```python
from build123d import *

# Parameters (mm, degrees)
CROQUIS2_R                 = 12.5
CROQUIS2_R_2               = 9.5
SALIENTE_EXTRUIR1_DEPTH    = 24
CORTAR_EXTRUIR3_DEPTH      = 191.437747955
CORTAR_EXTRUIR3_DEPTH_BACK = 191.437747955
CROQUIS5_W                 = 8
CROQUIS5_H                 = 49.434743854
CORTAR_EXTRUIR4_DEPTH      = 191.437747955
CORTAR_EXTRUIR4_DEPTH_BACK = 191.437747955
CROQUIS6_W                 = 12
CROQUIS6_H                 = 30
CORTAR_EXTRUIR5_DEPTH      = 159.265939688
CORTAR_EXTRUIR5_DEPTH_BACK = 159.265939688
CROQUIS7_W                 = 14.533349016
CROQUIS7_H                 = 8
REDONDEO1_R                = 4


with BuildPart() as part:
    # Croquis2 → Saliente-Extruir1 (new body)
    # profile 1 of 4: a face of its own
    with BuildSketch(Plane.XY):
        with Locations((-37.533349016, 172.653405471)):
            Circle(CROQUIS2_R)
        with Locations((-37.533349016, 172.653405471)):
            Circle(CROQUIS2_R_2, mode=Mode.SUBTRACT)
    # profile 2 of 4: a face of its own
    with BuildSketch(Plane.XY):
        with BuildLine():
            Line((-12.5, 58.855421297), (-12.5, 0))
            ThreePointArc((-12.5, 0), (0, 12.5), (12.5, 0))
            Line((12.5, 0), (12.5, 115))
            ThreePointArc((12.5, 115), (0.265693313, 156.217157525), (-32.475079629, 184.08423706))
            ThreePointArc((-32.475079629, 184.08423706), (-27.057701844, 179.473289366), (-25.033349016, 172.653405471))
            ThreePointArc((-25.033349016, 172.653405471), (-30.713465121, 162.1777583), (-42.591618403, 161.222573883))
            ThreePointArc((-42.591618403, 161.222573883), (-27.406897086, 150.843693068), (-16.941222141, 135.718661617))
            ThreePointArc((-16.941222141, 135.718661617), (-17.037727548, 131.417260647), (-20.439743892, 128.783319041))
            Line((-20.439743892, 128.783319041), (-27.655370554, 127.214704549))
            ThreePointArc((-27.655370554, 127.214704549), (-17.155961879, 124.732474812), (-12.5, 115))
            ThreePointArc((-12.5, 115), (-16.161165235, 106.161165235), (-25, 102.5))
            Line((-25, 102.5), (-17.5, 102.5))
            ThreePointArc((-17.5, 102.5), (-13.964466094, 101.035533906), (-12.5, 97.5))
            Line((-12.5, 97.5), (-12.5, 58.855421297))
        make_face()
    # profile 3 of 4: a face of its own
    with BuildSketch(Plane.XY):
        with Locations((-25, 115)):
            Circle(CROQUIS2_R)
        with Locations((-25, 115)):
            Circle(CROQUIS2_R_2, mode=Mode.SUBTRACT)
    # profile 4 of 4: a face of its own
    with BuildSketch(Plane.XY):
        Circle(CROQUIS2_R)
        Circle(CROQUIS2_R_2, mode=Mode.SUBTRACT)
    extrude(amount=SALIENTE_EXTRUIR1_DEPTH)

    # Croquis5 → Cortar-Extruir3 (cut, two sides: drawn at the far end of the back side and taken through both)
    with BuildSketch(Plane.ZY.offset(12.5).offset(-CORTAR_EXTRUIR3_DEPTH_BACK)):
        with Locations((12, 160.436033544)):
            Rectangle(CROQUIS5_W, CROQUIS5_H)
    extrude(amount=CORTAR_EXTRUIR3_DEPTH + CORTAR_EXTRUIR3_DEPTH_BACK, mode=Mode.SUBTRACT)

    # Croquis6 → Cortar-Extruir4 (cut, two sides: drawn at the far end of the back side and taken through both)
    with BuildSketch(Plane.ZY.offset(12.5).offset(-CORTAR_EXTRUIR4_DEPTH_BACK)):
        with Locations((12, 2.5)):
            Rectangle(CROQUIS6_W, CROQUIS6_H)
    extrude(amount=CORTAR_EXTRUIR4_DEPTH + CORTAR_EXTRUIR4_DEPTH_BACK, mode=Mode.SUBTRACT)

    # Croquis7 → Cortar-Extruir5 (cut, two sides: drawn at the far end of the back side and taken through both)
    with BuildSketch(Plane(origin=(0, 135.718661617, 0), x_dir=(1, 0, 0), z_dir=(0, 1, 0)).offset(-CORTAR_EXTRUIR5_DEPTH_BACK)):
        with Locations((-42.766674508, -12)):
            Rectangle(CROQUIS7_W, CROQUIS7_H)
    extrude(amount=CORTAR_EXTRUIR5_DEPTH + CORTAR_EXTRUIR5_DEPTH_BACK, mode=Mode.SUBTRACT)

    # Redondeo1
    # the kernel refuses this fillet: 4 mm, written as the material it adds along each edge
    with BuildSketch(Plane(origin=(-26.941222141, 135.718661617, 16), x_dir=(0, 1, 0), z_dir=(1, 0, 0))) as redondeo1_piece_1_section:
        with BuildLine():
            CenterArc((REDONDEO1_R, -REDONDEO1_R), REDONDEO1_R, 90, 90)
            Line((0, -REDONDEO1_R), (-REDONDEO1_R * 0.02, -REDONDEO1_R))
            Line((-REDONDEO1_R * 0.02, -REDONDEO1_R), (-REDONDEO1_R * 0.02, REDONDEO1_R * 0.02))
            Line((-REDONDEO1_R * 0.02, REDONDEO1_R * 0.02), (REDONDEO1_R, REDONDEO1_R * 0.02))
            Line((REDONDEO1_R, REDONDEO1_R * 0.02), (REDONDEO1_R, 0))
        make_face()
    redondeo1_piece_1 = extrude(amount=46.544739715, mode=Mode.PRIVATE)
    redondeo1_piece_1 = redondeo1_piece_1 & Plane(origin=(-63.045397247, 115.0005, 15.097345218), x_dir=(0.9999999999780976, -6.618536910383344e-06, 0), z_dir=(0, 0, -1)) * Cylinder(75.545397249, 110, mode=Mode.PRIVATE)
    redondeo1_piece_1 = redondeo1_piece_1 - Plane(origin=(-63.045397247, 115.0005, 15.097345218), x_dir=(0.40466155096197987, 0.9144665270927335, 0), z_dir=(0, 0, -1)) * Cylinder(50.545397249, 110, mode=Mode.PRIVATE)
    add(redondeo1_piece_1)
    with BuildSketch(Plane(origin=(19.603517574, 135.718661617, 8), x_dir=(0, 0, 1), z_dir=(-1, 0, 0))) as redondeo1_piece_2_section:
        with BuildLine():
            CenterArc((REDONDEO1_R, REDONDEO1_R), REDONDEO1_R, 180, 90)
            Line((0, REDONDEO1_R), (-REDONDEO1_R * 0.02, REDONDEO1_R))
            Line((-REDONDEO1_R * 0.02, REDONDEO1_R), (-REDONDEO1_R * 0.02, -REDONDEO1_R * 0.02))
            Line((-REDONDEO1_R * 0.02, -REDONDEO1_R * 0.02), (REDONDEO1_R, -REDONDEO1_R * 0.02))
            Line((REDONDEO1_R, -REDONDEO1_R * 0.02), (REDONDEO1_R, 0))
        make_face()
    redondeo1_piece_2 = extrude(amount=46.544739715, mode=Mode.PRIVATE)
    redondeo1_piece_2 = redondeo1_piece_2 - Plane(origin=(-63.045397247, 115.0005, 8.902651886), x_dir=(0.40466155096197987, 0.9144665270927335, 0), z_dir=(0, 0, -1)) * Cylinder(50.545397249, 110, mode=Mode.PRIVATE)
    redondeo1_piece_2 = redondeo1_piece_2 & Plane(origin=(-63.045397247, 115.0005, 8.902651886), x_dir=(0.9999999999780976, -6.618536910383344e-06, 0), z_dir=(0, 0, -1)) * Cylinder(75.545397249, 110, mode=Mode.PRIVATE)
    add(redondeo1_piece_2)
    with BuildSketch(Plane(origin=(-12.5, 17.5, 6), x_dir=(0, 0, 1), z_dir=(1, 0, 0))) as redondeo1_piece_3:
        with BuildLine():
            CenterArc((REDONDEO1_R, REDONDEO1_R), REDONDEO1_R, 180, 90)
            Line((0, REDONDEO1_R), (-REDONDEO1_R * 0.02, REDONDEO1_R))
            Line((-REDONDEO1_R * 0.02, REDONDEO1_R), (-REDONDEO1_R * 0.02, -REDONDEO1_R * 0.02))
            Line((-REDONDEO1_R * 0.02, -REDONDEO1_R * 0.02), (REDONDEO1_R, -REDONDEO1_R * 0.02))
            Line((REDONDEO1_R, -REDONDEO1_R * 0.02), (REDONDEO1_R, 0))
        make_face()
    extrude(amount=25)
    with BuildSketch(Plane(origin=(12.5, 17.5, 18), x_dir=(0, -1, 0), z_dir=(-1, 0, 0))) as redondeo1_piece_4:
        with BuildLine():
            CenterArc((REDONDEO1_R, -REDONDEO1_R), REDONDEO1_R, 90, 90)
            Line((0, -REDONDEO1_R), (-REDONDEO1_R * 0.02, -REDONDEO1_R))
            Line((-REDONDEO1_R * 0.02, -REDONDEO1_R), (-REDONDEO1_R * 0.02, REDONDEO1_R * 0.02))
            Line((-REDONDEO1_R * 0.02, REDONDEO1_R * 0.02), (REDONDEO1_R, REDONDEO1_R * 0.02))
            Line((REDONDEO1_R, REDONDEO1_R * 0.02), (REDONDEO1_R, 0))
        make_face()
    extrude(amount=25)


solid = part.part
```
The model under review builds one solid part; all positions refer to its coordinate system, in mm. A direction names the side the tool comes from. Coordinates: 2 decimals unless noted, no trailing zeros. Write each loop counter-clockwise with the first axis right and the second up, starting at its lowest first coordinate (ties: lowest second). Pieces come first, ordered by that corner, then holes. Notation, with made-up numbers: (-20, 78.5) - (34, 78.5) arc R22 ccw to (34, 108.5) - close; hole circle Ø10 at (-2.5, 8.5). An arc over 180 degrees is marked (long way). Write item = value, one per line.
(1) For P1, Ø8, axis at x = -11, z = 17.5, coming from the -Y side; P2, Ø22, axis at x = -37.53, y = 172.65, coming from the +Z side; P3, Ø2, axis at x = -16, z = 10, coming from the -Y side; P4, Ø1.5, axis at x = -39, z = 16.5, coming from the +Y side, all flat-tipped, find the tip position at first contact; note any pin that passes through.
Result sheet:
P1 = -10.33
P2 = 24
P3 = 101.83
P4 = 185.13
(2) Machinability: for faces 5 (the face through (-21, 102.5, 12)), 6 (the face through (-20, 162, 16)), 7 (the face through (-24, 128.01, 11.83)), which of the approach directions +Z, -Z, +X, -X, +Y, -Y give a long, thin tool a straight path to every point of the face, cutting with its end or side? Answer none if there is none.
Result sheet:
face_5 = +Z, -Z, -X, -Y
face_6 = +X, -X, +Y
face_7 = +Z, -Z, -X
(3) For line 1 (Y direction, x = -24, z = 7.75); line 2 (Z direction, x = -27.5, y = 164); line 3 (X direction, y = 32.5, z = 20), list the stretches that pass through material, from the lowest coordinate up. Write a range as [from, to].
Result sheet:
line_1 = [102.5, 105.55], [124.45, 128.01], [147.1, 179.67]
line_2 = [0, 8], [16, 24]
line_3 = [-12.5, 12.5]
(4) Mouldability with a two-part tool opening along X and no side actions: class faces 1 (the face through (-27.591, 151.026, 3.249)), 2 (the face through (4.38, -8.43, 20.96)), 3 (the face through (-5, 9, 18)), 4 (the face through (12.5, 57, 12)) as pulls with the +X half, pulls with the -X half, needs draft (parallel to the pull), parting line crosses it, or undercut.
Result sheet:
face_1 = pulls with the -X half
face_2 = undercut
face_3 = needs draft
face_4 = pulls with the +X half
(5) Consider section A-A, the plane y = 3.5. Give the boundary of the cut face in (x, z).
Result sheet:
outline = (-12.5, 0) - (-8.83, 0) - (-8.83, 6) - (-12.5, 6) - close; (-12.5, 18) - (-8.83, 18) - (-8.83, 24) - (-12.5, 24) - close; (8.83, 0) - (12.5, 0) - (12.5, 6) - (8.83, 6) - close; (8.83, 18) - (12.5, 18) - (12.5, 24) - (8.83, 24) - close
(6) Consider section D-D, the plane z = 20.25. Give the boundary of the cut face in (x, y).
Result sheet:
outline = (-42.59, 161.22) arc R50.55 cw to (-16.94, 135.72) arc R5 cw to (-20.44, 128.78) - (-27.66, 127.21) arc R12.5 ccw to (-25, 102.5) - (-17.5, 102.5) arc R5 cw to (-12.5, 97.5) - (-12.5, 0) arc R12.5 ccw to (12.5, 0) - (12.5, 115) arc R75.55 ccw to (-32.48, 184.08) arc R12.5 ccw to start; hole circle Ø19 at (-37.53, 172.65); hole circle Ø19 at (-25, 115); hole circle Ø19 at (0, 0)
(7) Consider section C-C, the plane x = -45. Give the boundary of the cut face in (y, z), then the cut area to 3 significant figures.
Result sheet:
outline = (162.63, 0) - (166.78, 0) - (166.78, 8) - (162.63, 8) - close; (162.63, 16) - (166.78, 16) - (166.78, 24) - (162.63, 24) - close; (178.53, 0) - (182.68, 0) - (182.68, 8) - (178.53, 8) - close; (178.53, 16) - (182.68, 16) - (182.68, 24) - (178.53, 24) - close
area = 133 mm^2
(8) Consider section B-B, the plane x = 0. Give the boundary of the cut face in (y, z), then the cut area to 3 significant figures.
Result sheet:
outline = (-12.5, 0) - (-9.5, 0) - (-9.5, 6) - (-12.5, 6) - close; (-12.5, 18) - (-9.5, 18) - (-9.5, 24) - (-12.5, 24) - close; (9.5, 0) - (156.62, 0) - (156.62, 8) - (139.72, 8) arc R4 cw to (139.72, 16) - (156.62, 16) - (156.62, 24) - (9.5, 24) - (9.5, 18) - (13.5, 18) arc R4 cw to (17.5, 14) - (17.5, 10) arc R4 cw to (13.5, 6) - (9.5, 6) - close
area = 3,320 mm^2
